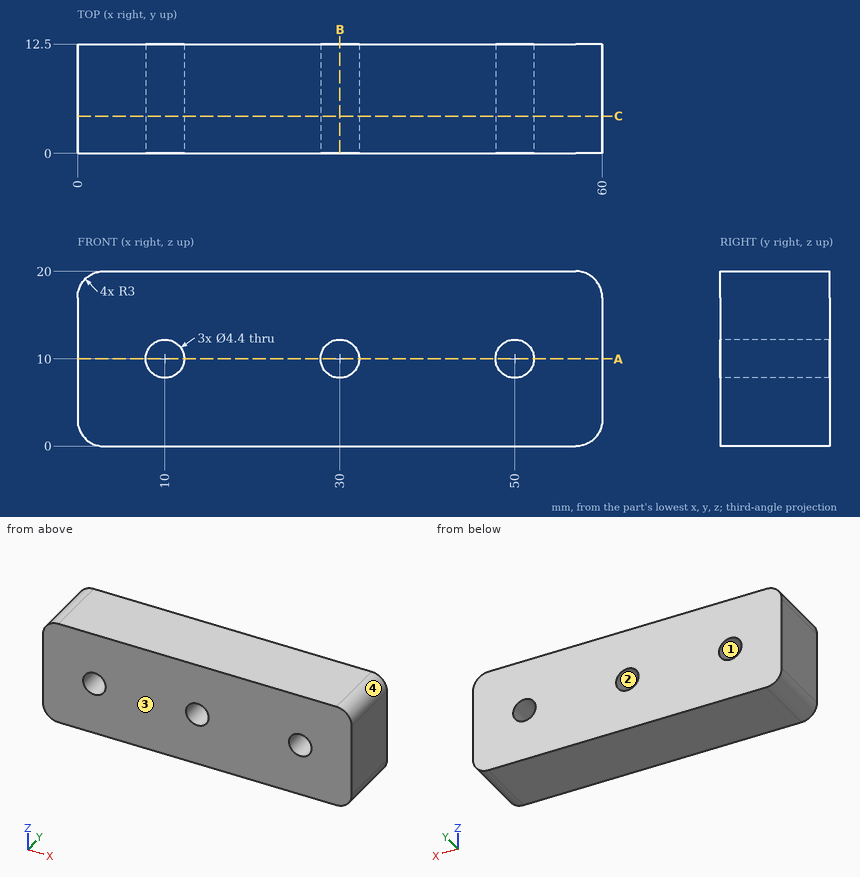
Here's the drawing with two shaded views (mm, measured from the low corner). I have some questions. Coordinates: 2 decimals unless noted, no trailing zeros. Loops run counter-clockwise (first coordinate to the right, second up) from the corner with the lowest first, then second, coordinate; pieces in that order, holes last. Notation, with made-up numbers: (-12.5, 39.5) -> (-4.5, 39.5) arc R32 ccw to (-4.5, 70.5) -> close; hole circle Ø2 at (25, -30). An arc over 180 degrees is marked (long way). Answer in a Markdown table with one row per item.
(1) Thinking about a two-plate mould opening in X: for the marked faces 1, 2, 3 and 4, which applies, released by +X, released by -X, zero draft, split by the parting line, or undercut?
Results found:
| item | result |
|---|---|
| face 1 | undercut |
| face 2 | undercut |
| face 3 | zero draft |
| face 4 | released by +X |
(2) If I drill on probe 1 along X at (y, z) = (5.75, 10); probe 2 along Z at (x, y) = (50, 5.75); probe 3 along X at (y, z) = (8.5, 10.75), over which ranges is the centre line in solid material (lowest first)?
Results found:
| item | result |
|---|---|
| probe 1 | x = 0 to 7.8, 12.2 to 27.8, 32.2 to 47.8, 52.2 to 60 |
| probe 2 | z = 0 to 7.8, 12.2 to 20 |
| probe 3 | x = 0 to 7.93, 12.07 to 27.93, 32.07 to 47.93, 52.07 to 60 |
(3) Imagine slicing it at B-B (x = 30). List the corners of the cut face in (y, z) for me.
Results found:
| item | result |
|---|---|
| outline | (0, 0) -> (12.5, 0) -> (12.5, 7.8) -> (0, 7.8) -> close; (0, 12.2) -> (12.5, 12.2) -> (12.5, 20) -> (0, 20) -> close |
(4) Imagine slicing it at C-C (y = 4.25). List the corners of the cut face in (x, z) for me.
Results found:
| item | result |
|---|---|
| outline | (0, 3) arc R3 ccw to (3, 0) -> (57, 0) arc R3 ccw to (60, 3) -> (60, 17) arc R3 ccw to (57, 20) -> (3, 20) arc R3 ccw to (0, 17) -> close; hole circle Ø4.4 at (10, 10); hole circle Ø4.4 at (30, 10); hole circle Ø4.4 at (50, 10) |
(5) Imagine slicing it at A-A (z = 10). List the corners of the cut face in (x, y) for me.
Results found:
| item | result |
|---|---|
| outline | (0, 0) -> (7.8, 0) -> (7.8, 12.5) -> (0, 12.5) -> close; (12.2, 0) -> (27.8, 0) -> (27.8, 12.5) -> (12.2, 12.5) -> close; (32.2, 0) -> (47.8, 0) -> (47.8, 12.5) -> (32.2, 12.5) -> close; (52.2, 0) -> (60, 0) -> (60, 12.5) -> (52.2, 12.5) -> close |
